CAD build for the part. Positions are in the model's coordinates, mm. Round coordinates to 2 decimals unless told otherwise and drop trailing zeros. Loops run counter-clockwise (first coordinate to the right, second up) from the corner with the lowest first, then second, coordinate; pieces in that order, holes last.
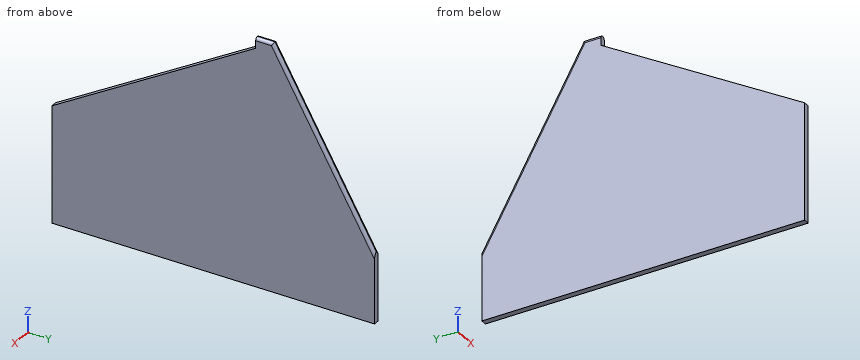
```python
from build123d import *

# Parameters (mm, degrees)
F0_W     = 113.7219756842
F0_H     = 120
F0_W_2   = 107.0308029652
F0_H_2   = 200
F1_DEPTH = 10
F2_R     = 4.99999


# Not quite as in the source:
# - a fillet or chamfer is up to 0.001 mm smaller than in the source, because OpenCascade refuses the exact size


with BuildPart() as f1:
    # F0 (on Right) → F1 (new body)
    with BuildSketch(Plane.YZ):
        with Locations((211.910609901, -14.3104368448)):
            Rectangle(F0_W, F0_H)
        Polygon((95.8531785295, -74.3104368448), (155.0496220589, -74.3104368448), (155.0496220589, 45.6895631552), (268.771597743, 45.6895631552), (95.8531785295, 349.9907631145), align=None)
        Polygon((66.0946071148, -74.3104368448), (95.8531785295, -74.3104368448), (95.8531785295, 349.9907631145), (66.0946071148, 332.2893329267), align=None)
        Polygon((66.0946071148, 332.2893329267), (95.8531785295, 349.9907631145), (66.0946071148, 349.9907631145), align=None)
        Polygon((-174.1975992918, -74.3104368448), (66.0946071148, -74.3104368448), (66.0946071148, 332.2893329267), (-281.228402257, 125.6895631552), (-174.1975992918, 125.6895631552), align=None)
        with Locations((-227.7130007744, 25.6895631552)):
            Rectangle(F0_W_2, F0_H_2)
    extrude(amount=F1_DEPTH)

    # F2 (radius 5 in the source; OpenCascade refuses exactly that, so slightly less here)
    f2_edges = [f1.edges().sort_by_distance(p)[0] for p in [
        (10, 182.312388, 197.840163),
        (0, 182.312388, 197.840163),
        (10, 80.973893, 349.990763),
        (0, 80.973893, 349.990763),
    ]]
    fillet(f2_edges, radius=F2_R)


solid = f1.part
```
Item 1: Cut at B-B, the plane y = -192. Give the cut face in (x, z).
Answers follow:
outline: (0, -74.31) - (10, -74.31) - (10, 178.77) - (0, 178.77) - close
Item 2: Cut at A-A, the plane x = 2.25. Give the cut face in (y, z).
Answers follow:
outline: (-281.23, -74.31) - (268.77, -74.31) - (268.77, 44.02) - (95.37, 349.17) - (66.09, 349.17) - (66.09, 332.29) - (-281.23, 125.69) - close
Item 3: Probe line 1 (Y direction, x = 3, z = 72); line 2 (Y direction, x = 4.75, z = 134); line 3 (Z direction, x = 5, y = -199.5). List the from-to ranges inside material, lowest first.
Answers follow:
line 1: y = -281.23 to 253.34
line 2: y = -267.26 to 218.58
line 3: z = -74.31 to 174.3
Item 4: Flat gauge pins, fed straight in: P1, Ø2, axis at x = 5.5, z = 247, coming from the -Y side; P2, Ø5, axis at x = 5.5, z = 342, coming from the -Y side. Where does each tip first touch, or does it go through?
Answers follow:
P1: stops at y = -78.97
P2: stops at y = 66.09
Item 5: Cut at C-C, the plane y = -126. Give the cut face in (x, z).
Answers follow:
outline: (0, -74.31) - (10, -74.31) - (10, 218.02) - (0, 218.02) - close
